Verification items for the finished model (mm, model axes). Face numbers are marked on the shaded views. A direction names the side the tool comes from. Coordinates: 2 decimals unless noted, no trailing zeros. Order: outer loops, then holes, each group sorted by start corner. A loop starts at its lowest first (then second) coordinate and runs counter-clockwise, first axis right, second up. Notation, with made-up numbers: M 26,-40 L 82,-40 A18 cw 82,-34 Z; hole C 60,12 d9. An arc over 180 degrees is marked long. Return JSON: item names as keys, results as strings. Group by question number.
1. Material ranges on line 1 along Z through (x, y) = (10, 9); line 2 along X through (y, z) = (0.25, -11.5); line 3 along Y through (x, z) = (-2.5, 1), recorded low to high.
2. Section check B-B, the plane z = -8. Record the cut outline in (x, y), plus the area to 3 significant figures.
3. Set-up check for the marked faces 1, 2 and 3: record each of +Z, -Z, +X, -X, +Y, -Y from which the full face is reachable in a straight line by a thin tool's end or side.
4. Section check A-A, the plane y = 0. Record the cut outline in (x, z).
5. Section check D-D, the plane y = 12.75. Record the cut outline in (x, z), plus the area to 3 significant figures.
6. Gauge pin test, flat ends, axial feed: pin 1 (2.5 mm diameter, centred on y = -1.5, z = 4, fed in from -X); pin 2 (10 mm diameter, centred on x = 9, y = 0, fed in from +Z); pin 3 (3 mm diameter, centred on x = -10.5, z = -1, fed in from -Y); pin 4 (2.5 mm diameter, centred on y = 2.5, z = 4.5, fed in from +X). Record the tip position at first contact, or that the pin passes through.
7. Section check C-C, the plane x = 11. Record the cut outline in (y, z).
```python
from build123d import *

# Parameters (mm, degrees)
BOSS_EXTRUDE2_DEPTH = 9.3


with BuildPart() as part:
    # Sketch6 → Boss-Extrude2 (new body)
    with BuildSketch(Plane.XY):
        Polygon((0, 10.68097998), (-9.25, 5.34048999), (-9.25, -5.34048999), (0, -10.68097998), (9.25, -5.34048999), (9.25, 5.34048999), align=None)
    extrude(amount=BOSS_EXTRUDE2_DEPTH)

    # Sketch8 → Cut-Revolve1 (revolve, cut)
    with BuildSketch(Plane(origin=(0, 0, 0), x_dir=(0, 0, -1), z_dir=(1, 0, 0)), mode=Mode.PRIVATE) as cut_revolve1_sk:
        Polygon((-7.3, 10.68097998), (-9.3, 8.68097998), (-9.3, 10.68097998), align=None)
    revolve(cut_revolve1_sk.sketch.rotate(Axis((0, 0, 0), (0, 0, 1)), 90), axis=Axis((0, 0, 0), (0, 0, 1)), mode=Mode.SUBTRACT)

    # Sketch10 → Revolve1 (revolve)
    with BuildSketch(Plane(origin=(0, 0, 0), x_dir=(0, 0, -1), z_dir=(1, 0, 0))):
        Polygon((0, 0), (0, 14.863694745), (3.2, 14.863694745), (3.2, 6.35), (30.851471863, 6.35), (31.7, 5.501471863), (31.7, 0), align=None)
    revolve(axis=Axis((0, 0, -31.7), (0, 0, 1)))


solid = part.part
```
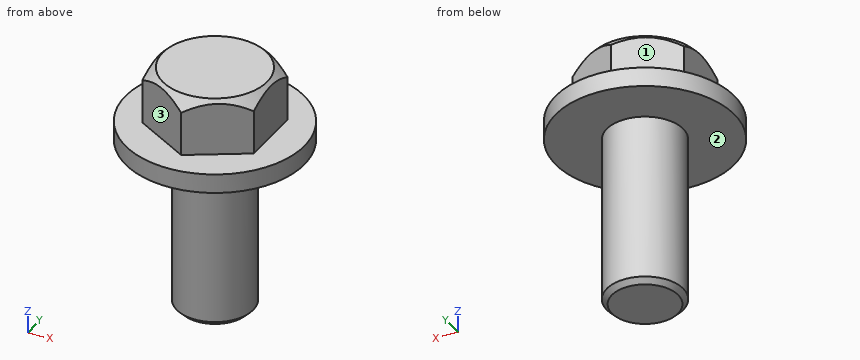
Answers follow:
{
 "1": {"line 1": "-3.2 to 0", "line 2": "-6.35 to 6.35", "line 3": "-9.24 to 9.24"},
 "2": {"outline": "C 0,0 d12.7", "area": "127 mm^2"},
 "3": {"face 1": "+Z, -X, +Y", "face 2": "-Z", "face 3": "+Z, -X, -Y"},
 "4": {"outline": "M -14.86,-3.2 L -6.35,-3.2 L -6.35,-30.85 L -5.5,-31.7 L 5.5,-31.7 L 6.35,-30.85 L 6.35,-3.2 L 14.86,-3.2 L 14.86,0 L 9.25,0 L 9.25,8.73 L 8.68,9.3 L -8.68,9.3 L -9.25,8.73 L -9.25,0 L -14.86,0 Z"},
 "5": {"outline": "M -7.64,-3.2 L 7.64,-3.2 L 7.64,0 L -7.64,0 Z", "area": "48.9 mm^2"},
 "6": {"pin 1": "x = -9.25", "pin 2": "z = 9.3", "pin 3": "y = -11.83", "pin 4": "x = 9.25"},
 "7": {"outline": "M -10,-3.2 L 10,-3.2 L 10,0 L -10,0 Z"}
}
